```python
from build123d import *

# Parameters (mm, degrees)
BOSS_EXTRUDE1_DEPTH = 9.899999946


with BuildPart() as part:
    # Sketch1 → Boss-Extrude1 (new body)
    with BuildSketch(Plane.XY.offset(9.899999946)):
        Polygon((14.973999709, 9.973499775), (14.973999709, 15.026499293), (30.026500597, 15.026499293), (30.026500597, 9.973499775), (25.026499852, 9.973499775), (25.026499852, 0), (34.999999627, 0), (34.999999627, 25), (25.026499852, 25), (25.026499852, 19.974000454), (19.973499403, 19.974000454), (19.973499403, 25), (9.999999627, 25), (9.999999627, 0), (19.973499403, 0), (19.973499403, 9.973499775), align=None)
    extrude(amount=-BOSS_EXTRUDE1_DEPTH)


solid = part.part
```
Source: CAD feature listing. Evaluate the final solid. Frame: model axes, mm. A direction names the side the tool comes from. Round coordinates to 2 decimals unless told otherwise and drop trailing zeros. Loops run counter-clockwise (first coordinate to the right, second up) from the corner with the lowest first, then second, coordinate; pieces in that order, holes last. Notation, with made-up numbers: M -8.75,-12.75 L 18.25,-12.75 A18 ccw 18.25,5.25 Z; hole C 69,26.25 d3. An arc over 180 degrees is marked long. Put each result on its own line as item: value.
(1) Section D-D, the plane x = 23.75. Return loops of the section in (y, z).
Solutions:
outline: M 15.03,0 L 19.97,0 L 19.97,9.9 L 15.03,9.9 Z
(2) Section A-A, the plane x = 19.5. Return loops of the section in (y, z), and give its area (3 significant figures).
Solutions:
outline: M 0,0 L 9.97,0 L 9.97,9.9 L 0,9.9 Z; M 15.03,0 L 25,0 L 25,9.9 L 15.03,9.9 Z
area: 197 mm²
(3) Section C-C, the plane z = 5.5. Return loops of the section in (x, y).
Solutions:
outline: M 10,0 L 19.97,0 L 19.97,9.97 L 14.97,9.97 L 14.97,15.03 L 30.03,15.03 L 30.03,9.97 L 25.03,9.97 L 25.03,0 L 35,0 L 35,25 L 25.03,25 L 25.03,19.97 L 19.97,19.97 L 19.97,25 L 10,25 Z
(4) Pull-direction query (Y, two-part tool) for faces 5 (the face through (14.974, 12, 5)), 6 (the face through (19.973, 22, 5)), 7 (the face through (30, 0, 5)); classes: released by +Y, released by -Y, zero draft, split by the parting line, or undercut.
Solutions:
face 5: undercut
face 6: zero draft
face 7: released by -Y
(5) Ray query, line 1 (Y direction, x = 29, z = 2.75); line 2 (X direction, y = 1, z = 1.25); line 3 (X direction, y = 12, z = 5.5). Return the intervals inside material, ascending. Write a range as [from, to].
Solutions:
line 1: [0, 9.97], [15.03, 25]
line 2: [10, 19.97], [25.03, 35]
line 3: [10, 14.97], [30.03, 35]
(6) Section B-B, the plane y = 22. Return loops of the section in (x, z), and give its area (3 significant figures).
Solutions:
outline: M 10,0 L 19.97,0 L 19.97,9.9 L 10,9.9 Z; M 25.03,0 L 35,0 L 35,9.9 L 25.03,9.9 Z
area: 197 mm²
(7) First-contact query: pin 1 (1.5 mm diameter, centred on x = 21.5, z = 5, fed in from +Y). Flat tip, straight axial feed; report the tip coordinate or a pass-through.
Solutions:
pin 1: y = 19.97
(8) Access query for faces 1 (the face through (15, 25, 5)), 2 (the face through (23, 19.974, 5)), 3 (the face through (25.026, 5, 5)), 4 (the face through (30.027, 13, 5)). Directions: +Z, -Z, +X, -X, +Y, -Y. A direction counts if a zero-diameter tool reaches every point of the face in a straight line with its end or side. Return the directions, or none.
Solutions:
face 1: +Z, -Z, +X, -X, +Y
face 2: +Z, -Z, +Y
face 3: +Z, -Z, -Y
face 4: +Z, -Z
